Input: part model. Units: mm. Frame: model coordinates. A direction names the side the tool comes from. Coordinates: 2 decimals unless noted, no trailing zeros. Order: outer loops, then holes, each group sorted by start corner. A loop starts at its lowest first (then second) coordinate and runs counter-clockwise, first axis right, second up.
from build123d import *

# Parameters (mm, degrees)
SKETCH1_R           = 0.75
SKETCH1_R_2         = 0.5
BOSS_EXTRUDE1_DEPTH = 2


with BuildPart() as part:
    # Sketch1 → Boss-Extrude1 (new body)
    with BuildSketch(Plane.XY):
        with BuildLine():
            Line((0, 6), (0, 11.795))
            ThreePointArc((0, 11.795), (1.464466094, 15.330533906), (5, 16.795))
            Line((5, 16.795), (11.2, 16.795))
            ThreePointArc((11.2, 16.795), (14.735533906, 15.330533906), (16.2, 11.795))
            Line((16.2, 11.795), (16.2, 6))
            Line((16.2, 6), (12.2, 6))
            Line((12.2, 6), (12.2, 4))
            Line((12.2, 4), (16.2, 4))
            Line((16.2, 4), (16.2, 2))
            ThreePointArc((16.2, 2), (15.614213562, 0.585786438), (14.2, 0))
            Line((14.2, 0), (2, 0))
            ThreePointArc((2, 0), (0.585786438, 0.585786438), (0, 2))
            Line((0, 2), (0, 4))
            Line((0, 4), (4, 4))
            Line((4, 4), (4, 6))
            Line((4, 6), (0, 6))
        make_face()
        with Locations((13.45, 2)):
            Circle(SKETCH1_R, mode=Mode.SUBTRACT)
        with Locations((13.45, 8)):
            Circle(SKETCH1_R, mode=Mode.SUBTRACT)
        with Locations((3, 13.795)):
            Circle(SKETCH1_R_2, mode=Mode.SUBTRACT)
        with Locations((13.2, 13.795)):
            Circle(SKETCH1_R_2, mode=Mode.SUBTRACT)
        with Locations((2.75, 8)):
            Circle(SKETCH1_R, mode=Mode.SUBTRACT)
        with Locations((2.75, 2)):
            Circle(SKETCH1_R, mode=Mode.SUBTRACT)
    extrude(amount=BOSS_EXTRUDE1_DEPTH)


solid = part.part
Item 1: Cut plane A-A on y = 8. Return loops of the section in (x, z).
Response values:
outline: (0, 0) - (2, 0) - (2, 2) - (0, 2) - close; (3.5, 0) - (12.7, 0) - (12.7, 2) - (3.5, 2) - close; (14.2, 0) - (16.2, 0) - (16.2, 2) - (14.2, 2) - close
Item 2: Cut plane C-C on z = 0.55. Return loops of the section in (x, y) (3 decimals), then the cut area to 3 significant figures.
Response values:
outline: (0, 2) arc R2 ccw to (2, 0) - (14.2, 0) arc R2 ccw to (16.2, 2) - (16.2, 4) - (12.2, 4) - (12.2, 6) - (16.2, 6) - (16.2, 11.795) arc R5 ccw to (11.2, 16.795) - (5, 16.795) arc R5 ccw to (0, 11.795) - (0, 6) - (4, 6) - (4, 4) - (0, 4) - close; hole circle Ø1.5 at (2.75, 2); hole circle Ø1.5 at (2.75, 8); hole circle Ø1 at (3, 13.795); hole circle Ø1.5 at (13.45, 2); hole circle Ø1.5 at (13.45, 8); hole circle Ø1 at (13.2, 13.795)
area: 235 mm2
Item 3: Ray query, probe 1 along X at (y, z) = (1.5, 0.45); probe 2 along Y at (x, z) = (2.75, 1.4); probe 3 along Y at (x, z) = (2.25, 0.45). Return the intervals inside material, ascending.
Response values:
probe 1: x = 0.06 to 2.19, 3.31 to 12.89, 14.01 to 16.14
probe 2: y = 0 to 1.25, 2.75 to 4, 6 to 7.25, 8.75 to 13.36, 14.23 to 16.26
probe 3: y = 0 to 1.44, 2.56 to 4, 6 to 7.44, 8.56 to 15.97
Item 4: Cut plane D-D on y = 14. Return loops of the section in (x, z).
Response values:
outline: (0.51, 0) - (2.54, 0) - (2.54, 2) - (0.51, 2) - close; (3.46, 0) - (12.74, 0) - (12.74, 2) - (3.46, 2) - close; (13.66, 0) - (15.69, 0) - (15.69, 2) - (13.66, 2) - close
Item 5: Cut plane B-B on x = 13.45. Return loops of the section in (y, z), then the cut area to 3 significant figures.
Response values:
outline: (0, 0) - (1.25, 0) - (1.25, 2) - (0, 2) - close; (2.75, 0) - (4, 0) - (4, 2) - (2.75, 2) - close; (6, 0) - (7.25, 0) - (7.25, 2) - (6, 2) - close; (8.75, 0) - (13.36, 0) - (13.36, 2) - (8.75, 2) - close; (14.23, 0) - (16.26, 0) - (16.26, 2) - (14.23, 2) - close
area: 20.8 mm2
Item 6: Access query for faces 5 (the face through (2, 4, 1)), 6 (the face through (8, 9, 2)), 7 (the face through (14, 6, 1)). Directions: +Z, -Z, +X, -X, +Y, -Y. A direction counts if a zero-diameter tool reaches every point of the face in a straight line with its end or side. Return the directions, or none.
Response values:
face 5: +Z, -Z, -X
face 6: +Z, +X, -X, +Y, -Y
face 7: +Z, -Z, +X
Item 7: Draft query along X for faces 1 (the face through (16.2, 9, 1)), 2 (the face through (1.426, 15.291, 0.986)), 3 (the face through (2, 6, 1)), 4 (the face through (14.165, 8.225, 0.986)). Return one class per face: pulls with the +X half, pulls with the -X half, needs draft (parallel to the pull), parting line crosses it, or undercut.
Response values:
face 1: pulls with the +X half
face 2: pulls with the -X half
face 3: needs draft
face 4: undercut
Item 8: Pin query (flat end, axial travel): pin 1 Ø1.4 at (x, y) = (2.75, 2) entering from -Z. Return the tip coordinate at first contact, or that it passes through.
Response values:
pin 1: passes through
